```python
from build123d import *

# Parameters (mm, degrees)
RESSALTO_EXTRUS_O1_DEPTH = 100
RESSALTO_EXTRUS_O3_REACH = 107.835
ESBO_O3_W                = 45
ESBO_O3_H                = 1.5
CORTE_EXTRUS_O1_DEPTH    = 103.343783397
ESBO_O5_W                = 12
ESBO_O5_H                = 1.5
CORTE_EXTRUS_O2_DEPTH    = 106.834776893
ESBO_O6_W                = 45
ESBO_O6_H                = 2
RESSALTO_EXTRUS_O4_DEPTH = 25
ESBO_O7_W                = 2.8
ESBO_O7_H                = 2.8
CORTE_EXTRUS_O3_DEPTH    = 10
CORTE_EXTRUS_O4_DEPTH    = 104.788245963
RESSALTO_EXTRUS_O5_DEPTH = 100
ESBO_O10_W               = 0.5
ESBO_O10_H               = 8
CORTE_EXTRUS_O5_DEPTH    = 104.788245963
CHANFRO1_SIZE            = 3
CHANFRO2_SIZE            = 3
RESSALTO_EXTRUS_O6_DEPTH = 100
CORTE_EXTRUS_O6_DEPTH    = 105.556204981
ESBO_O13_W               = 41
ESBO_O13_H               = 97.00005
CORTE_EXTRUS_O7_DEPTH    = 105.967852222
ESBO_O14_W               = 41
ESBO_O14_H               = 16
RESSALTO_EXTRUS_O7_DEPTH = 1


with BuildPart() as part:
    # Esboço1 → Ressalto-extrusão1 (new body)
    with BuildSketch(Plane.XY):
        Polygon((-22.5, 12.5), (-22.5, -7.5), (-17.5, -12.5), (17.5, -12.5), (22.5, -7.5), (22.5, 12.5), (24, 12.5), (24, -9), (19, -14), (-19, -14), (-24, -9), (-24, 12.5), align=None)
    extrude(amount=RESSALTO_EXTRUS_O1_DEPTH)

    # Ressalto-extrusão3: up to this face of the body (flat: up to its plane)
    ressalto_extrus_o3_end = Plane(part.part.faces().sort_by_distance((-23.25, 12.5, 50))[0])
    # Esboço3 → Ressalto-extrusão3 (add, up to the picked face)
    with BuildSketch(Plane(origin=(0, -12.5, 0), x_dir=(1, 0, 0), z_dir=(0, 1, 0)), mode=Mode.PRIVATE) as ressalto_extrus_o3_sk1:
        with Locations((0, -0.75)):
            Rectangle(ESBO_O3_W, ESBO_O3_H)
    ressalto_extrus_o3_tool1 = split(extrude(ressalto_extrus_o3_sk1.sketch, amount=RESSALTO_EXTRUS_O3_REACH, mode=Mode.PRIVATE), bisect_by=ressalto_extrus_o3_end, keep=Keep.BOTH, mode=Mode.PRIVATE)
    add(ressalto_extrus_o3_tool1.solids().sort_by(Axis((0, -12.5, 0.75), (0, 1, 0)))[0])

    # Esboço4 → Corte-extrusão1 (cut, through all)
    with BuildSketch(Plane.XY.offset(1.5)):
        Polygon((-10, -12.5), (10, -12.5), (10, -7.5), (5, -2.5), (-5, -2.5), (-10, -7.5), align=None)
    extrude(amount=-CORTE_EXTRUS_O1_DEPTH, mode=Mode.SUBTRACT)

    # Esboço5 → Corte-extrusão2 (cut, through all)
    with BuildSketch(Plane(origin=(0, -12.5, 0), x_dir=(1, 0, 0), z_dir=(0, 1, 0))):
        with Locations((0, -2.25)):
            Rectangle(ESBO_O5_W, ESBO_O5_H)
    extrude(amount=-CORTE_EXTRUS_O2_DEPTH, mode=Mode.SUBTRACT)

    # Esboço6 → Ressalto-extrusão4 (add)
    with BuildSketch(Plane(origin=(0, -12.5, 0), x_dir=(1, 0, 0), z_dir=(0, 1, 0))):
        with Locations((0, -99)):
            Rectangle(ESBO_O6_W, ESBO_O6_H)
    extrude(amount=RESSALTO_EXTRUS_O4_DEPTH)

    # Esboço7 → Corte-extrusão3 (cut)
    with BuildSketch(Plane.XY.offset(100)):
        with Locations((-8, 8.5)):
            Rectangle(ESBO_O7_W, ESBO_O7_H)
        with Locations((-16, 8.5)):
            Rectangle(ESBO_O7_W, ESBO_O7_H)
        with Locations((0, 8.5)):
            Rectangle(ESBO_O7_W, ESBO_O7_H)
        with Locations((8, 8.5)):
            Rectangle(ESBO_O7_W, ESBO_O7_H)
        with Locations((16, 8.5)):
            Rectangle(ESBO_O7_W, ESBO_O7_H)
        with Locations((-8, 0.5)):
            Rectangle(ESBO_O7_W, ESBO_O7_H)
        with Locations((0, 0.5)):
            Rectangle(ESBO_O7_W, ESBO_O7_H)
        with Locations((8, 0.5)):
            Rectangle(ESBO_O7_W, ESBO_O7_H)
        with Locations((16, 0.5)):
            Rectangle(ESBO_O7_W, ESBO_O7_H)
        with Locations((-8, -7.5)):
            Rectangle(ESBO_O7_W, ESBO_O7_H)
        with Locations((0, -7.5)):
            Rectangle(ESBO_O7_W, ESBO_O7_H)
        with Locations((8, -7.5)):
            Rectangle(ESBO_O7_W, ESBO_O7_H)
        with Locations((16, -7.5)):
            Rectangle(ESBO_O7_W, ESBO_O7_H)
        with Locations((-16, 0.5)):
            Rectangle(ESBO_O7_W, ESBO_O7_H)
        with Locations((-16, -7.5)):
            Rectangle(ESBO_O7_W, ESBO_O7_H)
    extrude(amount=-CORTE_EXTRUS_O3_DEPTH, mode=Mode.SUBTRACT)

    # Esboço8 → Corte-extrusão4 (cut, through all)
    with BuildSketch(Plane(origin=(0, 0, 0), x_dir=(-1, 0, 0), z_dir=(0, 0, -1))):
        Polygon((-22.5, -10.5), (-22.5, -12.5), (-20.5, -12.5), align=None)
        Polygon((20.5, -12.5), (22.5, -12.5), (22.5, -10.5), align=None)
    extrude(amount=-CORTE_EXTRUS_O4_DEPTH, mode=Mode.SUBTRACT)

    # Esboço9 → Ressalto-extrusão5 (add, through all)
    with BuildSketch(Plane(origin=(0, 0, 0), x_dir=(-1, 0, 0), z_dir=(0, 0, -1))):
        Polygon((-19, -14), (-21.5, -14), (-21.5, -11.5), align=None)
        Polygon((19, -14), (21.5, -14), (21.5, -11.5), align=None)
    extrude(amount=-RESSALTO_EXTRUS_O5_DEPTH)

    # Esboço10 → Corte-extrusão5 (cut, through all)
    with BuildSketch(Plane(origin=(0, 0, 0), x_dir=(-1, 0, 0), z_dir=(0, 0, -1))):
        with Locations((-23.75, 0.5)):
            Rectangle(ESBO_O10_W, ESBO_O10_H)
        with Locations((23.75, 0.5)):
            Rectangle(ESBO_O10_W, ESBO_O10_H)
    extrude(amount=-CORTE_EXTRUS_O5_DEPTH, mode=Mode.SUBTRACT)

    # Chanfro1
    # the kernel refuses this chamfer: 3 mm, written as the material it adds along each edge
    with BuildSketch(Plane(origin=(22.5, -15.215048964, 98), x_dir=(0.027495876610586768, 0, -0.9996219169112968), z_dir=(0, 1, 0))) as chanfro1_piece_1_section:
        Polygon((CHANFRO1_SIZE * 0.999621916911, CHANFRO1_SIZE * 0.0274958766106), (-CHANFRO1_SIZE * 0.0274958766106, CHANFRO1_SIZE * 0.999621916911), (0, 0), align=None)
    chanfro1_piece_1 = extrude(amount=27.715048964, mode=Mode.PRIVATE)
    chanfro1_piece_1 = split(chanfro1_piece_1, bisect_by=Plane(origin=(27.146986971, -2.853013029, 96.73534202), z_dir=(-0.7071067811865475, 0.7071067811865476, 0)), keep=Keep.TOP, mode=Mode.PRIVATE)
    add(chanfro1_piece_1)
    with BuildSketch(Plane(origin=(12.04463656, -17.95536344, 98), x_dir=(-0.7068394360706735, 0.7068394360706735, 0.027495876610586778), z_dir=(0.7071067811865476, 0.7071067811865475, 0))) as chanfro1_piece_2_section:
        Polygon((CHANFRO1_SIZE * 0.999621916911, -CHANFRO1_SIZE * 0.0274958766106), (-CHANFRO1_SIZE * 0.0274958766106, -CHANFRO1_SIZE * 0.999621916911), (0, 0), align=None)
    chanfro1_piece_2 = extrude(amount=22.50116574, mode=Mode.PRIVATE)
    chanfro1_piece_2 = split(chanfro1_piece_2, bisect_by=Plane(origin=(16.362312496, -12.5, 97.266244129), z_dir=(0, 1, 0)), keep=Keep.TOP, mode=Mode.PRIVATE)
    chanfro1_piece_2 = split(chanfro1_piece_2, bisect_by=Plane(origin=(16.362312496, -8.9, 97.266244129), z_dir=(0, -1, 0)), keep=Keep.TOP, mode=Mode.PRIVATE)
    add(chanfro1_piece_2)
    with BuildSketch(Plane(origin=(12.04463656, -17.95536344, 98), x_dir=(-0.7068394360706735, 0.7068394360706735, 0.027495876610586778), z_dir=(0.7071067811865476, 0.7071067811865475, 0))) as chanfro1_piece_3_section:
        Polygon((CHANFRO1_SIZE * 0.999621916911, -CHANFRO1_SIZE * 0.0274958766106), (-CHANFRO1_SIZE * 0.0274958766106, -CHANFRO1_SIZE * 0.999621916911), (0, 0), align=None)
    chanfro1_piece_3 = extrude(amount=22.50116574, mode=Mode.PRIVATE)
    chanfro1_piece_3 = split(chanfro1_piece_3, bisect_by=Plane(origin=(22.5, -7.314063038, 97.124733651), z_dir=(-1, 0, 0)), keep=Keep.TOP, mode=Mode.PRIVATE)
    chanfro1_piece_3 = split(chanfro1_piece_3, bisect_by=Plane(origin=(17.4, -7.314063038, 97.124733651), z_dir=(1, 0, 0)), keep=Keep.TOP, mode=Mode.PRIVATE)
    add(chanfro1_piece_3)
    with BuildSketch(Plane(origin=(25.215048964, -12.5, 98), x_dir=(0, -0.02749587661058619, -0.9996219169112968), z_dir=(-1, 0, 0))) as chanfro1_piece_4_section:
        Polygon((CHANFRO1_SIZE * 0.999621916911, -CHANFRO1_SIZE * 0.0274958766106), (-CHANFRO1_SIZE * 0.0274958766106, -CHANFRO1_SIZE * 0.999621916911), (0, 0), align=None)
    chanfro1_piece_4 = extrude(amount=50.430097928, mode=Mode.PRIVATE)
    chanfro1_piece_4 = split(chanfro1_piece_4, bisect_by=Plane(origin=(-9.263513514, -20.736486486, 97.013513514), z_dir=(0.7071067811865475, 0.7071067811865476, 0)), keep=Keep.TOP, mode=Mode.PRIVATE)
    chanfro1_piece_4 = split(chanfro1_piece_4, bisect_by=Plane(origin=(9.263513514, -20.736486486, 97.013513514), z_dir=(-0.7071067811865475, 0.7071067811865476, 0)), keep=Keep.TOP, mode=Mode.PRIVATE)
    add(chanfro1_piece_4)
    with BuildSketch(Plane(origin=(-27.95536344, -2.04463656, 98), x_dir=(0.7068394360706733, 0.7068394360706736, 0.027495876610586757), z_dir=(0.7071067811865476, -0.7071067811865475, 0))) as chanfro1_piece_5_section:
        Polygon((CHANFRO1_SIZE * 0.999621916911, -CHANFRO1_SIZE * 0.0274958766106), (-CHANFRO1_SIZE * 0.0274958766106, -CHANFRO1_SIZE * 0.999621916911), (0, 0), align=None)
    chanfro1_piece_5 = extrude(amount=22.50116574, mode=Mode.PRIVATE)
    chanfro1_piece_5 = split(chanfro1_piece_5, bisect_by=Plane(origin=(-22.5, -3.439339828, 97.957106781), z_dir=(1, 0, 0)), keep=Keep.TOP, mode=Mode.PRIVATE)
    chanfro1_piece_5 = split(chanfro1_piece_5, bisect_by=Plane(origin=(-17.4, -3.439339828, 97.957106781), z_dir=(-1, 0, 0)), keep=Keep.TOP, mode=Mode.PRIVATE)
    add(chanfro1_piece_5)
    with BuildSketch(Plane(origin=(-27.95536344, -2.04463656, 98), x_dir=(0.7068394360706733, 0.7068394360706736, 0.027495876610586757), z_dir=(0.7071067811865476, -0.7071067811865475, 0))) as chanfro1_piece_6_section:
        Polygon((CHANFRO1_SIZE * 0.999621916911, -CHANFRO1_SIZE * 0.0274958766106), (-CHANFRO1_SIZE * 0.0274958766106, -CHANFRO1_SIZE * 0.999621916911), (0, 0), align=None)
    chanfro1_piece_6 = extrude(amount=22.50116574, mode=Mode.PRIVATE)
    chanfro1_piece_6 = split(chanfro1_piece_6, bisect_by=Plane(origin=(-16.362312496, -12.5, 97.266244129), z_dir=(0, 1, 0)), keep=Keep.TOP, mode=Mode.PRIVATE)
    chanfro1_piece_6 = split(chanfro1_piece_6, bisect_by=Plane(origin=(-16.362312496, -8.9, 97.266244129), z_dir=(0, -1, 0)), keep=Keep.TOP, mode=Mode.PRIVATE)
    add(chanfro1_piece_6)
    with BuildSketch(Plane(origin=(-22.5, -15.215048964, 98), x_dir=(-0.027495876610586768, 0, -0.9996219169112968), z_dir=(0, 1, 0))) as chanfro1_piece_7_section:
        Polygon((CHANFRO1_SIZE * 0.999621916911, -CHANFRO1_SIZE * 0.0274958766106), (-CHANFRO1_SIZE * 0.0274958766106, -CHANFRO1_SIZE * 0.999621916911), (0, 0), align=None)
    chanfro1_piece_7 = extrude(amount=27.715048964, mode=Mode.PRIVATE)
    chanfro1_piece_7 = split(chanfro1_piece_7, bisect_by=Plane(origin=(-27.146986971, -2.853013029, 96.73534202), z_dir=(0.7071067811865475, 0.7071067811865476, 0)), keep=Keep.TOP, mode=Mode.PRIVATE)
    add(chanfro1_piece_7)

    # Chanfro2
    chanfro2_edges = [part.edges().sort_by_distance(p)[0] for p in [
        (-13.75, -12.5, 1.5),
        (20, -10, 1.5),
        (-22.5, 2.5, 1.5),
        (-20, -10, 1.5),
        (22.5, 2.5, 1.5),
        (13.75, -12.5, 1.5),
    ]]
    chamfer(chanfro2_edges, length=CHANFRO2_SIZE)

    # Esboço12 → Corte-extrusão6 (cut, through all)
    with BuildSketch(Plane(origin=(0, 0, 0), x_dir=(-1, 0, 0), z_dir=(0, 0, -1))):
        Polygon((24, -9), (24, -3.5), (23.5, -3.5), (23.5, 4.5), (24, 4.5), (24, 12.5), (-24, 12.5), (-24, 4.5), (-23.5, 4.5), (-23.5, -3.5), (-24, -3.5), (-24, -9), (-21.5, -11.5), (-21.5, -14), (21.5, -14), (21.5, -11.5), align=None)
    extrude(amount=-CORTE_EXTRUS_O6_DEPTH, mode=Mode.SUBTRACT)


with BuildPart() as body_2:
    # Esboço11 → Ressalto-extrusão6 (new, through all)
    with BuildSketch(Plane(origin=(0, 0, 0), x_dir=(-1, 0, 0), z_dir=(0, 0, -1))):
        Polygon((24.5, -9.207106781), (24.5, -3), (24, -3), (24, 4), (26, 4), (26, -14.5), (26, -16), (-26, -16), (-26, -14.5), (-26, 4), (-24, 4), (-24, -3), (-24.5, -3), (-24.5, -9.207106781), (-22, -11.707106781), (-22, -14.5), (22, -14.5), (22, -11.707106781), align=None)
    extrude(amount=-RESSALTO_EXTRUS_O6_DEPTH)

    # Esboço13 → Corte-extrusão7 (cut, through all)
    with BuildSketch(Plane(origin=(0, -14.5, 0), x_dir=(1, 0, 0), z_dir=(0, 1, 0))):
        with Locations((0, -50.000025)):
            Rectangle(ESBO_O13_W, ESBO_O13_H)
    extrude(amount=-CORTE_EXTRUS_O7_DEPTH, mode=Mode.SUBTRACT)

    # Esboço14 → Ressalto-extrusão7 (add)
    with BuildSketch(Plane.XZ.offset(16)):
        with Locations((0, 82.00005)):
            Rectangle(ESBO_O14_W, ESBO_O14_H)
        with Locations((0, 18)):
            Rectangle(ESBO_O14_W, ESBO_O14_H)
    extrude(amount=-RESSALTO_EXTRUS_O7_DEPTH)


solid = body_2.part
```
Could you check a few things on this model? Use its own coordinates, in mm. A direction names the side the tool comes from. Round coordinates to 2 decimals unless told otherwise and drop trailing zeros. Write each loop counter-clockwise with the first axis right and the second up, starting at its lowest first coordinate (ties: lowest second). Pieces come first, ordered by that corner, then holes. Notation, with made-up numbers: M -2.75,-22.5 L 18.25,-22.5 A25 ccw 18.25,4.5 Z; hole C -4,61.25 d10. An arc over 180 degrees is marked long. Write each question's results on one line, items separated by ' | '. Start each with the question number.
1. Imagine slicing it at C-C on z = 66. List the corners of the cut face in (x, y) for me.
2. Thinking about a two-plate mould opening in X: for faces 4 (the face through (-25, 4, 49)), 5 (the face through (-21, -14.5, 50)), 6 (the face through (26, -6, 49)), which applies, +X half, -X half, draft (parallel to the pull), parting line (faces both ways), or undercut?
3. I need wall thicknesses on L1, parallel to X at y = 1.5, z = 25.5; L2, parallel to X at y = -12, z = 73.5; L3, parallel to Y at x = 14.5, z = 19. Which ranges of each line are inside material? Lowest first, please. Write a range as from..to.
4. Imagine slicing it at A-A on y = 0.25. List the corners of the cut face in (x, z) for me.
5. Imagine slicing it at D-D on z = 20. List the corners of the cut face in (x, y) for me.
6. I'm going to push a flat-ended pin straight in: pin 1 Ø17.5 at (x, z) = (4.5, 83) entering from +Y. Where does the tip first touch, or does it pass through?
7. On a 3-axis mill with a long thin cutter (end or side, diameter ignored), from which of +Z, -Z, +X, -X, +Y, -Y can I reach the whole of each face in a straight line? I mean faces 1 (the face through (-24.5, -6, 49)), 2 (the face through (0, -15, 18)), 3 (the face through (22, -13, 49)). Say none if no direction works.
8. Imagine slicing it at B-B on x = -19.5. List the corners of the cut face in (y, z) for me.
Result sheet:
1) outline: M -26,-16 L -20.5,-16 L -20.5,-14.5 L -22,-14.5 L -22,-11.71 L -24.5,-9.21 L -24.5,-3 L -24,-3 L -24,4 L -26,4 Z; M 20.5,-16 L 26,-16 L 26,4 L 24,4 L 24,-3 L 24.5,-3 L 24.5,-9.21 L 22,-11.71 L 22,-14.5 L 20.5,-14.5 Z
2) face 4: draft | face 5: undercut | face 6: +X half
3) L1: x = -26..-24, 24..26 | L2: x = -26..-22, 22..26 | L3: y = -16..-15
4) outline: M -26,0 L -24,0 L -24,100 L -26,100 Z; M 24,0 L 26,0 L 26,100 L 24,100 Z
5) outline: M -26,-16 L 26,-16 L 26,4 L 24,4 L 24,-3 L 24.5,-3 L 24.5,-9.21 L 22,-11.71 L 22,-14.5 L 20.5,-14.5 L 20.5,-15 L -20.5,-15 L -20.5,-14.5 L -22,-14.5 L -22,-11.71 L -24.5,-9.21 L -24.5,-3 L -24,-3 L -24,4 L -26,4 Z
6) pin 1: stops at y = -15
7) face 1: +Z, -Z | face 2: +Y | face 3: +Z, -Z, +Y
8) outline: M -16,0 L -14.5,0 L -14.5,1.5 L -16,1.5 Z; M -16,10 L -15,10 L -15,26 L -16,26 Z; M -16,74 L -15,74 L -15,90 L -16,90 Z; M -16,98.5 L -14.5,98.5 L -14.5,100 L -16,100 Z
